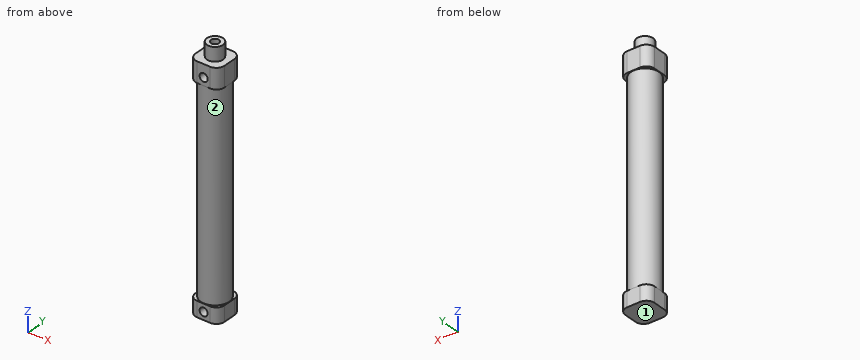
from build123d import *

# Parameters (mm, degrees)
SKETCH_1_W          = 18
SKETCH_1_H          = 18
EXTRUDE_1_DEPTH     = 9.5
SKETCH_2_R          = 8.75
EXTRUDE_2_DEPTH     = 125.5
SKETCH_3_W          = 18
SKETCH_3_H          = 18
EXTRUDE_3_DEPTH     = 12.5
SKETCH_4_R          = 5
EXTRUDE_4_DEPTH     = 8.5
SKETCH_5_R          = 2.5
CUT_EXTRUDE_1_DEPTH = 155
FILLET_1_R          = 5
CUT_EXTRUDE_2_REACH = 20
SKETCH_6_R          = 2.5


with BuildPart() as part:
    # 草图1 → 凸台-拉伸1 (new body)
    with BuildSketch(Plane.XY):
        Rectangle(SKETCH_1_W, SKETCH_1_H)
    extrude(amount=EXTRUDE_1_DEPTH)

    # 草图2 → 凸台-拉伸2 (add)
    with BuildSketch(Plane.XY.offset(9.5)):
        Circle(SKETCH_2_R)
    extrude(amount=EXTRUDE_2_DEPTH)

    # 草图3 → 凸台-拉伸3 (add)
    with BuildSketch(Plane.XY.offset(135)):
        Rectangle(SKETCH_3_W, SKETCH_3_H)
    extrude(amount=EXTRUDE_3_DEPTH)

    # 草图4 → 凸台-拉伸4 (add)
    with BuildSketch(Plane.XY.offset(147.5)):
        Circle(SKETCH_4_R)
    extrude(amount=EXTRUDE_4_DEPTH)

    # 草图5 → 切除-拉伸1 (cut)
    with BuildSketch(Plane.XY.offset(156)):
        Circle(SKETCH_5_R)
    extrude(amount=-CUT_EXTRUDE_1_DEPTH, mode=Mode.SUBTRACT)

    # 圆角1
    fillet_1_edges = [part.edges().sort_by_distance(p)[0] for p in [
        (9, -9, 141.25),
        (9, 9, 141.25),
        (-9, 9, 141.25),
        (-9, -9, 141.25),
        (9, -9, 4.75),
        (-9, -9, 4.75),
        (-9, 9, 4.75),
        (9, 9, 4.75),
    ]]
    fillet(fillet_1_edges, radius=FILLET_1_R)

    # 草图6 → 切除-拉伸2 (cut, up to next)
    with BuildSketch(Plane.XZ.offset(9), mode=Mode.PRIVATE) as cut_extrude_2_sk1:
        with Locations((0, 4.75)):
            Circle(SKETCH_6_R)
    cut_extrude_2_tool1 = extrude(cut_extrude_2_sk1.sketch, amount=-CUT_EXTRUDE_2_REACH, mode=Mode.PRIVATE) & part.part
    add(cut_extrude_2_tool1.solids().sort_by_distance((0, -9, 4.75))[0], mode=Mode.SUBTRACT)
    # 草图6 → 切除-拉伸2 (cut, up to next)
    with BuildSketch(Plane.XZ.offset(9), mode=Mode.PRIVATE) as cut_extrude_2_sk2:
        with Locations((0, 139.75)):
            Circle(SKETCH_6_R)
    cut_extrude_2_tool2 = extrude(cut_extrude_2_sk2.sketch, amount=-CUT_EXTRUDE_2_REACH, mode=Mode.PRIVATE) & part.part
    add(cut_extrude_2_tool2.solids().sort_by_distance((0, -9, 139.75))[0], mode=Mode.SUBTRACT)


solid = part.part
Verification items for the finished model (mm, model axes). Face numbers are marked on the shaded views. Coordinates: 2 decimals unless noted, no trailing zeros. Write each loop counter-clockwise with the first axis right and the second up, starting at its lowest first coordinate (ties: lowest second). Pieces come first, ordered by that corner, then holes. Notation, with made-up numbers: (30, -37.5) - (80, -37.5) arc R34 cw to (80, 1.5) - close; hole circle Ø1 at (23.25, 56). An arc over 180 degrees is marked (long way). Answer as a JSON object with one key per item and string values.
(1) Mould release check, pull along Z, two halves, no side actions. Record for the marked faces 1 and 2: pulls with the +Z half, pulls with the -Z half, needs draft (parallel to the pull), parting line crosses it, or undercut.
Report:
{"face 1": "pulls with the -Z half", "face 2": "undercut"}
(2) Cross-section at B-B on z = 4.75. Record the cut outline in (x, y).
Report:
{"outline": "(-9, -4) arc R5 ccw to (-4, -9) - (-2.5, -9) - (-2.5, 0) arc R2.5 cw to (2.5, 0) - (2.5, -9) - (4, -9) arc R5 ccw to (9, -4) - (9, 4) arc R5 ccw to (4, 9) - (-4, 9) arc R5 ccw to (-9, 4) - close"}
(3) Gauge pin test, flat ends, axial feed: pin 1 Ø6 at (x, z) = (-3.5, 52) entering from +Y; pin 2 Ø4 at (x, z) = (-7, 130) entering from +Y; pin 3 Ø1.5 at (y, z) = (3, 71) entering from -X. Record the tip position at first contact, or that the pin passes through.
Report:
{"pin 1": "y = 8.74", "pin 2": "y = 7.18", "pin 3": "x = -8.46"}
(4) Cross-section at A-A on x = 0. Record the cut outline in (y, z).
Report:
{"outline": "(-9, 0) - (9, 0) - (9, 9.5) - (8.75, 9.5) - (8.75, 135) - (9, 135) - (9, 147.5) - (5, 147.5) - (5, 156) - (2.5, 156) - (2.5, 1) - (-2.5, 1) - (-2.5, 2.25) - (-9, 2.25) - close; (-9, 7.25) - (-2.5, 7.25) - (-2.5, 137.25) - (-9, 137.25) - (-9, 135) - (-8.75, 135) - (-8.75, 9.5) - (-9, 9.5) - close; (-9, 142.25) - (-2.5, 142.25) - (-2.5, 156) - (-5, 156) - (-5, 147.5) - (-9, 147.5) - close"}
(5) Thickness scan on line 1 along Z through (x, y) = (0, -6); line 2 along Z through (x, y) = (0, -2.75); line 3 along X through (y, z) = (-4.25, 139.75). Record the ranges inside material, lowest first.
Report:
{"line 1": "0 to 2.25, 7.25 to 137.25, 142.25 to 147.5", "line 2": "0 to 2.25, 7.25 to 137.25, 142.25 to 156", "line 3": "-8.99 to -2.5, 2.5 to 8.99"}
(6) Cross-section at C-C on z = 28.5. Record the cut outline in (x, y).
Report:
{"outline": "circle Ø17.5 at (0, 0); hole circle Ø5 at (0, 0)"}
